```python
from build123d import *

# Parameters (mm, degrees)
CROQUIS1_W              = 21
CROQUIS1_H              = 15
SALIENTE_EXTRUIR1_DEPTH = 13.5
CROQUIS2_W              = 21
CROQUIS2_H              = 15
CROQUIS2_W_2            = 18.9
CROQUIS2_H_2            = 12.9
CORTAR_EXTRUIR1_DEPTH   = 10.5
SALIENTE_EXTRUIR2_DEPTH = 5.25
REDONDEO1_R             = 0.5
CROQUIS4_W              = 1.418006124
CROQUIS4_H              = 6.039970015
CROQUIS4_H_2            = 6.039970016
SALIENTE_EXTRUIR3_DEPTH = 10.5


with BuildPart() as part:
    # Croquis1 → Saliente-Extruir1 (new body)
    with BuildSketch(Plane.XY):
        Rectangle(CROQUIS1_W, CROQUIS1_H)
    extrude(amount=SALIENTE_EXTRUIR1_DEPTH)

    # Croquis2 → Cortar-Extruir1 (cut)
    with BuildSketch(Plane.XY.offset(13.5)):
        Rectangle(CROQUIS2_W, CROQUIS2_H)
        Rectangle(CROQUIS2_W_2, CROQUIS2_H_2, mode=Mode.SUBTRACT)
    extrude(amount=-CORTAR_EXTRUIR1_DEPTH, mode=Mode.SUBTRACT)

    # Croquis3 → Saliente-Extruir2 (add, symmetric)
    with BuildSketch(Plane(origin=(0, 0, 0), x_dir=(1, 0, 0), z_dir=(0, 1, 0))):
        with BuildLine():
            Line((7.039280928, 0), (-7.963522393, 0))
            add(Edge.make_bspline(
                [(-5.706653699, 3.481138081), (-7.057942912, 2.763187698), (-7.488467217, 1.307416204), (-7.963522393, 0)],
                knots=[0, 0, 0, 0, 1, 1, 1, 1], degree=3))
            add(Edge.make_bspline(
                [(7.039280928, 0), (4.224020061, 0.069217615), (-0.214677684, 0.66683062), (-4.502921069, 2.204677744), (-5.706653699, 3.481138081)],
                knots=[0, 0, 0, 0, 0.62405833, 1, 1, 1, 1], degree=3))
        make_face()
    extrude(amount=SALIENTE_EXTRUIR2_DEPTH, both=True)

    # Redondeo1
    redondeo1_edges = [part.edges().sort_by_distance(p)[0] for p in [
        (-5.706653699, -2.625, -3.481138081),
    ]]
    fillet(redondeo1_edges, radius=REDONDEO1_R)

    # Croquis4 → Saliente-Extruir3 (add)
    with BuildSketch(Plane.XY.offset(13.5)):
        with Locations((-7.552748408, -0.069775705)):
            Rectangle(CROQUIS4_W, CROQUIS4_H)
        with Locations((-0.194042943, -0.039922945)):
            Rectangle(CROQUIS4_W, CROQUIS4_H)
        with Locations((6.78276327, -0.08977409)):
            Rectangle(CROQUIS4_W, CROQUIS4_H_2)
    extrude(amount=SALIENTE_EXTRUIR3_DEPTH)


solid = part.part
```
Design review of the part built by this model. Coordinates are the model's own, in mm. A direction names the side the tool comes from. Give positions to 0.01 mm unless a question says otherwise; leave off trailing zeros. Loops run counter-clockwise (first coordinate to the right, second up) from the corner with the lowest first, then second, coordinate; pieces in that order, holes last. Notation, with made-up numbers: M 19,-33 L 72,-33 A16 cw 72,-18 Z; hole C 29,74 d9. An arc over 180 degrees is marked long. Return JSON: item names as keys, results as strings. Group by question number.
Item 1: We need section C-C (z = 6). Give the boundary of the cut face in (x, y), and give its area (3 significant figures).
Item 2: We need section A-A (z = 16.75). Give the boundary of the cut face in (x, y).
Item 3: Tool access review of faces 4 (the flat face through (-6.844, 0, 19)), 5 (the flat face through (-4, 5.25, -1)), 6 (the flat face through (7, 2.93, 19)), 7 (the flat face through (-8.262, 0, 19)): name each direction out of +Z, -Z, +X, -X, +Y, -Y from which nothing blocks a thin tool from reaching the whole face with its end or side.
Item 4: We need section B-B (x = 9). Give the boundary of the cut face in (y, z).
Item 5: For probe 1 along X at (y, z) = (-1, 22.75); probe 2 along Y at (x, z) = (-9.25, 10.5); probe 3 along Y at (x, z) = (-7, 22.75), list the stretches that pass through material, from the lowest coordinate up.
Item 6: Insertion check: pin 1 Ø3 at (y, z) = (2.5, 9) entering from +X; pin 2 Ø5 at (x, z) = (-0.5, 8) entering from -Y; pin 3 Ø1.1 at (x, z) = (0, 16.5) entering from -Y. Each pin has a flat end and moves straight along its axis. Give the tip position at first contact, or say it passes through.
Item 7: Mouldability with a two-part tool opening along X and no side actions: class faces 1 (the flat face through (-0.903, 0, 19)), 2 (the flat face through (0, 0, 24)), 3 (the flat face through (9.45, 0, 8)) as released by +X, released by -X, zero draft, split by the parting line, or undercut.
Output:
{
 "1": {"outline": "M -9.45,-6.45 L 9.45,-6.45 L 9.45,6.45 L -9.45,6.45 Z", "area": "244 mm^2"},
 "2": {"outline": "M -8.26,-3.09 L -6.84,-3.09 L -6.84,2.95 L -8.26,2.95 Z; M -0.9,-3.06 L 0.51,-3.06 L 0.51,2.98 L -0.9,2.98 Z; M 6.07,-3.11 L 7.49,-3.11 L 7.49,2.93 L 6.07,2.93 Z"},
 "3": {"face 4": "+Z, +Y, -Y", "face 5": "-Z, +X, -X, +Y", "face 6": "+Z, +X, +Y", "face 7": "+Z, -X, +Y, -Y"},
 "4": {"outline": "M -7.5,0 L 7.5,0 L 7.5,3 L 6.45,3 L 6.45,13.5 L -6.45,13.5 L -6.45,3 L -7.5,3 Z"},
 "5": {"probe 1": "x = -8.26 to -6.84, -0.9 to 0.51, 6.07 to 7.49", "probe 2": "y = -6.45 to 6.45", "probe 3": "y = -3.09 to 2.95"},
 "6": {"pin 1": "stops at x = 9.45", "pin 2": "stops at y = -6.45", "pin 3": "stops at y = -3.06"},
 "7": {"face 1": "undercut", "face 2": "zero draft", "face 3": "released by +X"}
}
